Autodesk Inventor part; units mm, degrees
ref_plane "YZ Plane" through (0, 0, 0) normal (1, 0, 0) x (0, 1, 0)
ref_plane "XZ Plane" through (0, 0, 0) normal (0, 1, 0) x (-1, 0, 0)
ref_plane "XY Plane" through (0, 0, 0) normal (0, 0, 1) x (1, 0, 0)
sketch "Sketch1" plane through (0, 0, 0) normal (0, 1, 0) x (-1, 0, 0)
  line L0 (5, 2.8868) -> (5, -2.8868)
  line L1 (5, -2.8868) -> (0, -5.7735)
  line L2 (0, -5.7735) -> (-5, -2.8868)
  line L3 (-5, -2.8868) -> (-5, 2.8868)
  line L4 (-5, 2.8868) -> (0, 5.7735)
  line L5 (0, 5.7735) -> (5, 2.8868)
  point P0 (0, 0)
  point P1 (0, 0)
  dimension "d0" = 10
extrude "Extrusion1" add sketch "Sketch1" along normal blind 6
sketch "Sketch2" plane through (0, 6, 0) normal (0, 1, 0) x (1, 0, 0)
  point P0 (0, 0)
  point P1 (0, 0)
hole "Hole1" at (0, 6, 0) direction (0, -1, 0) diameter 4.917 end through all
sketch "Sketch3" plane through (0, 0, 0) normal (1, 0, 0) x (0, 1, 0)
  line L0 (0, 0) -> (9.121, 0)
  line L1 (0, 5.7735) -> (6, 5.7735)
  line L2 (2.5, 5.7735) -> (1.7265, 5)
  line L3 (1.7265, 5) -> (0, 5)
  line L4 (0, 5) -> (0, 5.7735)
  line L5 (6, 5.7735) -> (6, 2.8868)
  dimension "d10" = 10
  dimension "d11" = 3.5
  dimension "d12" = 45
revolve "Revolution1" cut sketch "Sketch3" angle 360 about axis through (0, 0, 0) along (0, 1, 0)
fillet "Fillet1" radius 0.5 1 edges at (0, 0, -5)
sketch "Sketch4" plane through (0, 0, 0) normal (0, -1, 0) x (1, 0, 0)
  circle A0 centre (0, 0) radius 4.5
  circle A1 centre (0, 0) radius 3.75
  dimension "d15" = 7.5
split_face "Split1"
sketch "Sketch5" plane through (0, 0, 0) normal (1, 0, 0) x (0, 1, 0)
  line L0 (0, 0) -> (10.6904, 0)
  line L1 (2.5, 5.7735) -> (6, 5.7735)
  line L2 (5, 5.7735) -> (6, 5)
  line L3 (6, 5) -> (6, 5.7735)
  line L4 (6, 5) -> (10.4328, 5)
  dimension "d16" = 1
  dimension "d17" = 10
revolve "Revolution2" cut sketch "Sketch5" angle 360 about axis through (0, 0, 0) along (0, 1, 0)
chamfer "Chamfer1" distance 0.5 angle 45 1 edges at (0, 6, -2.4585)
properties part number "M6 nyloc" material "Steel, Carbon"
The model under review builds one solid part; all positions refer to its coordinate system, in mm. Give positions to 0.01 mm unless a question says otherwise; leave off trailing zeros. Loops run counter-clockwise (first coordinate to the right, second up) from the corner with the lowest first, then second, coordinate; pieces in that order, holes last. Notation, with made-up numbers: (69.25, 9) - (96.25, 9) arc R21 cw to (96.25, 45) - close; hole circle Ø4 at (-1.5, 30.5). An arc over 180 degrees is marked (long way). Answer as a JSON object with one key per item and string values.
Q1. Insertion check: pin 1 (3 mm diameter, centred on x = 0, z = 0, fed in from +Y); pin 2 (3 mm diameter, centred on x = 3, y = 2, fed in from +Z). Each pin has a flat end and moves straight along its axis. Give the tip position at first contact, or say it passes through.
Worked out:
{"pin 1": "passes through", "pin 2": "stops at z = 4.91"}
Q2. To check wall thickness, follow line 1 along X through (y, z) = (3.55, 0); line 2 along Z through (x, y) = (2.5, 3.1); line 3 along X through (y, z) = (0.35, 1.75). State the ranges of each line that lie inside material, in increasing order.
Worked out:
{"line 1": "x = -5 to -2.46, 2.46 to 5", "line 2": "z = -4.33 to 4.33", "line 3": "x = -4.66 to -1.73, 1.73 to 4.66"}
Q3. Add section B-B on y = 4.1. State the section outline as (x, z) points.
Worked out:
{"outline": "(-5, -2.89) - (0, -5.77) - (5, -2.89) - (5, 2.89) - (0, 5.77) - (-5, 2.89) - close; hole circle Ø4.92 at (0, 0)"}
Q4. Mouldability with a two-part tool opening along Z and no side actions: class faces 1 (the conical face through (4.487, 1.915, 2.605)), 2 (the conical face through (4.487, 5.757, -2.605)), 3 (the cylindrical face through (-0.738, 2.712, 2.345)) as +Z half, -Z half, draft (parallel to the pull), parting line (faces both ways), or undercut.
Worked out:
{"face 1": "+Z half", "face 2": "-Z half", "face 3": "undercut"}
Q5. Add section A-A on y = 2.25. State the section outline as (x, z) points.
Worked out:
{"outline": "(-5, -2.35) arc R5.52 ccw to (-4.53, -3.16) - (-0.47, -5.5) arc R5.52 ccw to (0.47, -5.5) - (4.53, -3.16) arc R5.52 ccw to (5, -2.35) - (5, 2.35) arc R5.52 ccw to (4.53, 3.16) - (0.47, 5.5) arc R5.52 ccw to (-0.47, 5.5) - (-4.53, 3.16) arc R5.52 ccw to (-5, 2.35) - close; hole circle Ø4.92 at (0, 0)"}
